from build123d import *
from build123d.topology import SkipClean

# Parameters (mm, degrees)
SKETCH1_W           = 20
SKETCH1_H           = 20
BOSS_EXTRUDE1_DEPTH = 2
SKETCH3_R           = 2.5
CUT_EXTRUDE1_DEPTH  = 15.282857
SKETCH4_W           = 12
SKETCH4_H           = 12
CUT_EXTRUDE2_DEPTH  = 1
SKETCH5_W           = 2
SKETCH5_H           = 20
BOSS_EXTRUDE2_DEPTH = 38
CUT_EXTRUDE3_DEPTH  = 46.825757
SKETCH7_R           = 10
BOSS_EXTRUDE3_DEPTH = 7.5
BOSS_EXTRUDE4_START = -7.5
SKETCH8_R           = 10
BOSS_EXTRUDE4_DEPTH = 7.5
CUT_EXTRUDE4_DEPTH  = 46.825757
CUT_EXTRUDE5_DEPTH  = 46.825757
FILLET1_R           = 5
FILLET2_R           = 5
FILLET3_R           = 5
FILLET4_R           = 5


with BuildPart() as part:
    # Sketch1 → Boss-Extrude1 (new body)
    with BuildSketch(Plane.XY):
        Rectangle(SKETCH1_W, SKETCH1_H)
    extrude(amount=BOSS_EXTRUDE1_DEPTH)

    # Sketch3 → Cut-Extrude1 (cut, through all)
    with BuildSketch(Plane(origin=(0, 0, 0), x_dir=(-1, 0, 0), z_dir=(0, 0, -1))):
        Circle(SKETCH3_R)
    extrude(amount=-CUT_EXTRUDE1_DEPTH, mode=Mode.SUBTRACT)

    # Sketch4 → Cut-Extrude2 (cut)
    with BuildSketch(Plane.XY.offset(2)):
        Rectangle(SKETCH4_W, SKETCH4_H)
    extrude(amount=-CUT_EXTRUDE2_DEPTH, mode=Mode.SUBTRACT)

    # Sketch5 → Boss-Extrude2 (add)
    with BuildSketch(Plane.XY.offset(2)):
        with Locations((9, 0)):
            Rectangle(SKETCH5_W, SKETCH5_H)
        with Locations((-9, 0)):
            Rectangle(SKETCH5_W, SKETCH5_H)
    extrude(amount=BOSS_EXTRUDE2_DEPTH)

    # Sketch6 → Cut-Extrude3 (cut, through all)
    with BuildSketch(Plane.ZY.offset(10)):
        with BuildLine():
            Line((40, 10), (30, 10))
            ThreePointArc((30, 10), (37.071068, 7.071068), (40, 0))
            Line((40, 0), (40, 10))
        make_face()
        with BuildLine():
            Line((40, -10), (40, 0))
            ThreePointArc((40, 0), (37.071068, -7.071068), (30, -10))
            Line((30, -10), (40, -10))
        make_face()
    extrude(amount=-CUT_EXTRUDE3_DEPTH, mode=Mode.SUBTRACT)

    # Sketch7 → Boss-Extrude3 (add)
    with SkipClean():  # the faces are left unmerged after this step: merging them gives an invalid solid
        with BuildSketch(Plane.ZY.offset(10)):
            with Locations((30, 0)):
                Circle(SKETCH7_R)
        extrude(amount=-BOSS_EXTRUDE3_DEPTH)

    # Sketch8 → Boss-Extrude4 (add)
    with SkipClean():  # the faces are left unmerged after this step: merging them gives an invalid solid
        with BuildSketch(Plane(origin=(10, 0, 0), x_dir=(0, 0, -1), z_dir=(1, 0, 0)).offset(BOSS_EXTRUDE4_START)):
            with Locations(Location((-30, 0, 0), (0, 0, 180))):
                Circle(SKETCH8_R)
        extrude(amount=BOSS_EXTRUDE4_DEPTH)

    # Sketch9 → Cut-Extrude4 (cut, through all)
    with SkipClean():  # the faces are left unmerged after this step: merging them gives an invalid solid
        with BuildSketch(Plane.ZY.offset(10)):
            with BuildLine():
                ThreePointArc((31.5, 4), (31.06066, 5.06066), (30, 5.5))
                Line((30, 5.5), (30, 2.5))
                ThreePointArc((30, 2.5), (31.06066, 2.93934), (31.5, 4))
            make_face()
            with BuildLine():
                Line((30, 2.5), (30, 5.5))
                ThreePointArc((30, 5.5), (28.5, 4), (30, 2.5))
            make_face()
            with BuildLine():
                ThreePointArc((31.5, -4), (31.06066, -2.93934), (30, -2.5))
                Line((30, -2.5), (30, -5.5))
                ThreePointArc((30, -5.5), (31.06066, -5.06066), (31.5, -4))
            make_face()
            with BuildLine():
                Line((30, -5.5), (30, -2.5))
                ThreePointArc((30, -2.5), (28.5, -4), (30, -5.5))
            make_face()
        extrude(amount=-CUT_EXTRUDE4_DEPTH, mode=Mode.SUBTRACT)

    # Sketch11 → Cut-Extrude5 (cut, through all)
    with SkipClean():  # the faces are left unmerged after this step: merging them gives an invalid solid
        with BuildSketch(Plane(origin=(10, 0, 0), x_dir=(0, 0, -1), z_dir=(1, 0, 0))):
            with BuildLine():
                Line((-30, -10), (-2, -10))
                Line((-2, -10), (-2, -5))
                Line((-2, -5), (-21.339746, -5))
                ThreePointArc((-21.339746, -5), (-25, -8.660254), (-30, -10))
            make_face()
            with BuildLine():
                Line((-2, 10), (-30, 10))
                ThreePointArc((-30, 10), (-25, 8.660254), (-21.339746, 5))
                Line((-21.339746, 5), (-2, 5))
                Line((-2, 5), (-2, 10))
            make_face()
        extrude(amount=-CUT_EXTRUDE5_DEPTH, mode=Mode.SUBTRACT)

    # Fillet1
    fillet1_edges = [part.edges().sort_by_distance(p)[0] for p in [
        (-10, 10, 1),
    ]]
    fillet(fillet1_edges, radius=FILLET1_R)

    # Fillet2
    fillet2_edges = [part.edges().sort_by_distance(p)[0] for p in [
        (10, 10, 1),
    ]]
    fillet(fillet2_edges, radius=FILLET2_R)

    # Fillet3
    fillet3_edges = [part.edges().sort_by_distance(p)[0] for p in [
        (10, -10, 1),
    ]]
    fillet(fillet3_edges, radius=FILLET3_R)

    # Fillet4
    fillet4_edges = [part.edges().sort_by_distance(p)[0] for p in [
        (-10, -10, 1),
    ]]
    fillet(fillet4_edges, radius=FILLET4_R)


solid = part.part
Verification items for the finished model (mm, model axes). A direction names the side the tool comes from. Give positions to 0.01 mm unless a question says otherwise; leave off trailing zeros. Write each loop counter-clockwise with the first axis right and the second up, starting at its lowest first coordinate (ties: lowest second). Pieces come first, ordered by that corner, then holes. Notation, with made-up numbers: M 20,-18 L 41,-18 A28 cw 41,20 Z; hole C 16.5,-31 d3. An arc over 180 degrees is marked long. Use CSV: the item, a comma, the result in double quotes.
1) Cross-section at D-D (x = 0). Enter the section's corners in (y, z).
Final values:
outline,"M -10,0 L -2.5,0 L -2.5,1 L -6,1 L -6,2 L -10,2 Z; M 2.5,0 L 10,0 L 10,2 L 6,2 L 6,1 L 2.5,1 Z"
2) Go/stop test with flat-tipped pins: pin 1 Ø1 at (x, z) = (9.5, 8) entering from -Y; pin 2 Ø5 at (x, z) = (-3, 35) entering from -Y; pin 3 Ø1 at (x, z) = (-6.5, 33.5) entering from +Y. Record where each tip stops, or that it passes through.
Final values:
pin 1,"y = -5"
pin 2,"y = -9.68"
pin 3,"y = 9.54"
3) Material ranges on line 1 along X through (y, z) = (-8.5, 30); line 2 along X through (y, z) = (-4, 3); line 3 along Z through (x, y) = (-7.75, 2.75), recorded low to high.
Final values:
line 1,"-10 to -2.5, 2.5 to 10"
line 2,"-10 to -8, 8 to 10"
line 3,"0 to 2, 20.39 to 29.17, 30.83 to 39.61"
4) Cross-section at C-C (y = 1). Enter the section's corners in (x, z), plus the area to 3 significant figures.
Final values:
outline,"M -10,0 L -2.29,0 L -2.29,1 L -6,1 L -6,2 L -8,2 L -8,20.05 L -2.5,20.05 L -2.5,39.95 L -10,39.95 Z; M 2.29,0 L 10,0 L 10,39.95 L 2.5,39.95 L 2.5,20.05 L 8,20.05 L 8,2 L 6,2 L 6,1 L 2.29,1 Z"
area,"394 mm²"
5) Access from +Z, -Z, +X, -X, +Y, -Y to the whole of each face (thin tool, end or side, straight path). Record for faces 1 (the face through (-2.5, 0, 30)), 2 (the face through (3, 0, 1)), 3 (the face through (-8, 9, 1)).
Final values:
face 1,"+Z, +Y, -Y"
face 2,"none"
face 3,"-Z, -X, +Y"
6) Release check for a two-part mould opening along Z. For faces 4 (the face through (2, 2, 0)), 5 (the face through (-0.1, -6, 1.5)), 6 (the face through (9, -8, 1)) record: released by +Z, released by -Z, zero draft, split by the parting line, or undercut.
Final values:
face 4,"released by -Z"
face 5,"undercut"
face 6,"zero draft"
7) Cross-section at B-B (z = 11). Enter the section's corners in (x, y).
Final values:
outline,"M -10,-5 L -8,-5 L -8,5 L -10,5 Z; M 8,-5 L 10,-5 L 10,5 L 8,5 Z"
8) Cross-section at A-A (x = -3). Enter the section's corners in (y, z), plus the area to 3 significant figures.
Final values:
outline,"M -10,0 L 10,0 L 10,2 L 6,2 L 6,1 L -6,1 L -6,2 L -10,2 Z; C 0,30 d20; hole C -4,30 d3; hole M 2.5,30 A1.5 ccw long 4,31.5 A1.5 ccw Z"
area,"328 mm²"
